Geometry check sheet. Reference: the model listing, model coordinates, mm. A direction names the side the tool comes from. Round coordinates to 2 decimals unless told otherwise and drop trailing zeros. Loops run counter-clockwise (first coordinate to the right, second up) from the corner with the lowest first, then second, coordinate; pieces in that order, holes last. Notation, with made-up numbers: M 37.25,-18 L 75.25,-18 A18 cw 75.25,-1 Z; hole C -25.75,13 d2. An arc over 180 degrees is marked long. Answer in a Markdown table with one row per item. Add a question column.
```python
from build123d import *

# Parameters (mm, degrees)
SKETCH_1_W      = 390
SKETCH_1_H      = 450
SKETCH_1_R      = 8
SKETCH_1_W_2    = 290
SKETCH_1_H_2    = 350
EXTRUDE_1_DEPTH = 15


with BuildPart() as part:
    # 草图1 → 凸台-拉伸1 (new body)
    with BuildSketch(Plane(origin=(0, 0, 0), x_dir=(0, 0, -1), z_dir=(1, 0, 0))):
        Rectangle(SKETCH_1_W, SKETCH_1_H)
        with Locations((-180, 175)):
            Circle(SKETCH_1_R, mode=Mode.SUBTRACT)
        with Locations(Location((-180, -175, 0), (0, 0, 180))):
            Circle(SKETCH_1_R, mode=Mode.SUBTRACT)
        with Locations((-180, 0)):
            Circle(SKETCH_1_R, mode=Mode.SUBTRACT)
        with Locations(Location((180, 175, 0), (0, 0, 180))):
            Circle(SKETCH_1_R, mode=Mode.SUBTRACT)
        with Locations(Location((180, 0, 0), (0, 0, 180))):
            Circle(SKETCH_1_R, mode=Mode.SUBTRACT)
        with Locations((180, -175)):
            Circle(SKETCH_1_R, mode=Mode.SUBTRACT)
        Rectangle(SKETCH_1_W_2, SKETCH_1_H_2, mode=Mode.SUBTRACT)
    extrude(amount=EXTRUDE_1_DEPTH)


solid = part.part
```
1) Cross-section at C-C, the plane y = 51.5. Record the boundary of the cut face in (x, z).
2) Cross-section at A-A, the plane y = 0. Record the boundary of the cut face in (x, z), plus the area to 3 significant figures.
3) Set-up check for faces 4 (the flat face through (7, -3, -195)), 5 (the flat face through (7, -2, -145)): record each of +Z, -Z, +X, -X, +Y, -Y from which the full face is reachable in a straight line by a thin tool's end or side.
4) Cross-section at B-B, the plane z = 180. Record the boundary of the cut face in (x, y).
5) Cross-section at D-D, the plane x = 12.75. Record the boundary of the cut face in (y, z).
6) Thickness scan on L1, parallel to Y at x = 3.5, z = -180; L2, parallel to Z at x = 6.75, y = 0.5; L3, parallel to Y at x = 1.5, z = -93.5. Record the ranges inside material, lowest first. Write a range as [from, to].
7) Draft check along Y on faces 1 (the cylindrical face through (7.4, -182.81, -178.27)), 2 (the flat face through (7, 225, 3)), 3 (the flat face through (7, -3, 195)). Enter one of: +Y half, -Y half, draft (parallel to the pull), parting line (faces both ways), or undercut.
Worked answers:
| question | item | result |
|---|---|---|
| 1 | outline | M 0,-195 L 15,-195 L 15,-145 L 0,-145 Z; M 0,145 L 15,145 L 15,195 L 0,195 Z |
| 2 | outline | M 0,-195 L 15,-195 L 15,-188 L 0,-188 Z; M 0,-172 L 15,-172 L 15,-145 L 0,-145 Z; M 0,145 L 15,145 L 15,172 L 0,172 Z; M 0,188 L 15,188 L 15,195 L 0,195 Z |
| 2 | area | 1,020 mm2 |
| 3 | face 4 | -Z, +X, -X, +Y, -Y |
| 3 | face 5 | +X, -X |
| 4 | outline | M 0,-225 L 15,-225 L 15,-183 L 0,-183 Z; M 0,-167 L 15,-167 L 15,-8 L 0,-8 Z; M 0,8 L 15,8 L 15,167 L 0,167 Z; M 0,183 L 15,183 L 15,225 L 0,225 Z |
| 5 | outline | M -225,-195 L 225,-195 L 225,195 L -225,195 Z; hole C -175,-180 d16; hole C -175,180 d16; hole M -175,-145 L 175,-145 L 175,145 L -175,145 Z; hole C 0,-180 d16; hole C 0,180 d16; hole C 175,-180 d16; hole C 175,180 d16 |
| 6 | L1 | y = [-225, -183], [-167, -8], [8, 167], [183, 225] |
| 6 | L2 | z = [-195, -187.98], [-172.02, -145], [145, 172.02], [187.98, 195] |
| 6 | L3 | y = [-225, -175], [175, 225] |
| 7 | face 1 | undercut |
| 7 | face 2 | +Y half |
| 7 | face 3 | draft |
